The listing builds one solid part. Answer for the finished solid, in the listing's coordinates (mm). Face numbers are marked on the shaded views. A direction names the side the tool comes from. Round coordinates to 2 decimals unless told otherwise and drop trailing zeros. Order: outer loops, then holes, each group sorted by start corner. A loop starts at its lowest first (then second) coordinate and runs counter-clockwise, first axis right, second up. Notation, with made-up numbers: (-35, -0.75) - (-19, -0.75) arc R10 ccw to (-19, 18.25) - close; hole circle Ø10 at (-2, 44). An arc over 180 degrees is marked (long way). Use CSV: the item, a comma, the result in double quotes. Start each with the question number.
Item 1: For the marked faces 1, 2 and 3, determine the directions among +Z, -Z, +X, -X, +Y, -Y from which every point of the face is accessible in a straight line to the end or side of a thin tool.
Item 2: Find section A-A, the plane y = 1.6. Give the vertices of the cut face in (x, z) (3 decimals).
Item 3: Find section B-B, the plane x = 2.55. Count the separate pieces of the cut face and the enclosed holes in it, plus the area to 3 significant figures.
Item 4: A flat-ended cylindrical pin translates along its axis: P1, Ø1.1, axis at x = 0.5, y = -1, coming from the -Z side. Find the tip coordinate at first contact, or state that the pin passes through.
Item 5: Determine the mould class of the marked faces 4, 5, 6 and 7 for opening direction X: +X half, -X half, draft (parallel to the pull), parting line (faces both ways), or undercut.
Item 6: Straight lines are drawn through the part: line 1 along Y through (x, z) = (-0.1, 2.5); line 2 along X through (y, z) = (-1.2, 4.5) (3 decimals); line 3 along Z through (x, y) = (0.8, -2.15). For each, find the intervals that lie inside material, in ascending order. Write a range as [from, to].
Item 7: Find section C-C, the plane z = 3.25. Give the vertices of the cut face in (x, y) (3 decimals).
```python
from build123d import *

# Parameters (mm, degrees)
SKETCH006_W      = 1.85
SKETCH006_H      = 1.4
EXTRUDE006_DEPTH = 6.3
SKETCH007_W      = 1
SKETCH007_H      = 1
EXTRUDE007_DEPTH = 9
SKETCH010_W      = 4
SKETCH010_H      = 4
EXTRUDE010_DEPTH = 0.5
SKETCH011_W      = 3.2
SKETCH011_H      = 5
EXTRUDE011_DEPTH = 6.8
CHAMFER002_SIZE  = 0.4
ARRAY004_X_COUNT = 2
ARRAY004_X_PITCH = 2.54


with BuildPart() as extrude006:
    # Sketch006 → Extrude006 (new body)
    with BuildSketch(Plane.XY):
        Rectangle(SKETCH006_W, SKETCH006_H)
    extrude(amount=EXTRUDE006_DEPTH)


with BuildPart() as fusion004:
    # Sketch007 → Extrude007 (new body)
    with BuildSketch(Plane.XY):
        Rectangle(SKETCH007_W, SKETCH007_H)
    extrude(amount=EXTRUDE007_DEPTH)

    # Fusion004: union Extrude006
    add(extrude006.part)


with BuildPart() as fusion004_1:
    # Fusion004 placement: moved
    add(fusion004.part.moved(Location((0, 1.27, 0))))


with BuildPart() as extrude010:
    # Sketch010 → Extrude010 (new body)
    with BuildSketch(Plane.XY):
        Rectangle(SKETCH010_W, SKETCH010_H)
    extrude(amount=EXTRUDE010_DEPTH)


with BuildPart() as fusion005:
    # Part__Mirroring002: instance of Fusion004
    add(fusion004_1.part.mirror(Plane(origin=(0, 0, 0), x_dir=(1, 0, 0), z_dir=(0, 1, 0))))

    # Fusion005: union Fusion004, Extrude010
    add(fusion004_1.part)
    add(extrude010.part)


with BuildPart() as body002:
    # Sketch011 → Extrude011 (new body)
    with BuildSketch(Plane.XY):
        Rectangle(SKETCH011_W, SKETCH011_H)
    extrude(amount=EXTRUDE011_DEPTH)

    # Cut: cut Fusion005
    add(fusion005.part, mode=Mode.SUBTRACT)

    # Chamfer002
    chamfer002_edges = [body002.edges().sort_by_distance(p)[0] for p in [
        (0, -0.77, 6.8),
        (-0.5, -1.27, 6.8),
        (0, -1.77, 6.8),
        (0.5, -1.27, 6.8),
        (0.5, 1.27, 6.8),
        (0, 1.77, 6.8),
        (-0.5, 1.27, 6.8),
        (0, 0.77, 6.8),
    ]]
    chamfer(chamfer002_edges, length=CHAMFER002_SIZE)

    # Array004 X: body002 ×2


with BuildPart() as body002_1:
    add(body002.part)
    with Locations(*[(i * ARRAY004_X_PITCH, 0, 0) for i in range(1, ARRAY004_X_COUNT)]):
        add(body002.part)


solid = body002_1.part
```
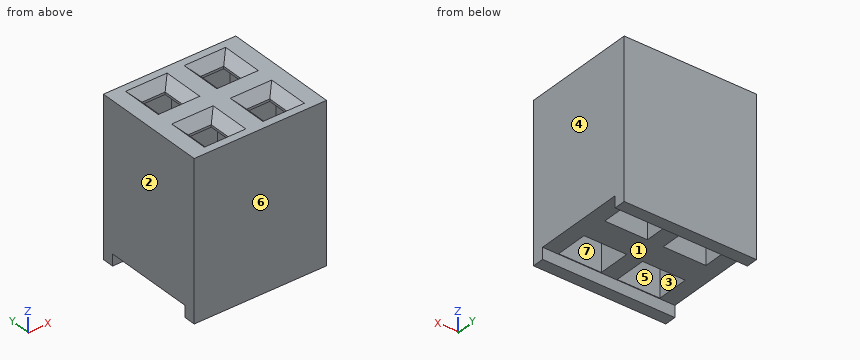
Worked out:
1,face 1,"-Z, +X, -X"
1,face 2,"+Z, -Z, -X, +Y, -Y"
1,face 3,"-Z"
2,outline,"(-1.6, 0.5) - (-0.925, 0.5) - (-0.925, 6.3) - (-0.5, 6.3) - (-0.5, 6.4) - (-0.9, 6.8) - (-1.6, 6.8) - close; (0.5, 6.3) - (0.925, 6.3) - (0.925, 0.5) - (1.615, 0.5) - (1.615, 6.3) - (2.04, 6.3) - (2.04, 6.4) - (1.64, 6.8) - (0.9, 6.8) - (0.5, 6.4) - close; (3.04, 6.3) - (3.465, 6.3) - (3.465, 0.5) - (4.14, 0.5) - (4.14, 6.8) - (3.44, 6.8) - (3.04, 6.4) - close"
3,separate pieces,"3"
3,enclosed holes,"0"
3,area,"14.4 mm²"
4,P1,"stops at z = 0.5"
5,face 4,"+X half"
5,face 5,"undercut"
5,face 6,"draft"
5,face 7,"undercut"
6,line 1,"y = [-2.5, -1.97], [-0.57, 0.57], [1.97, 2.5]"
6,line 2,"x = [-1.6, -0.925], [0.925, 1.615], [3.465, 4.14]"
6,line 3,"z = [0, 6.78]"
7,outline,"(-1.6, -2.5) - (4.14, -2.5) - (4.14, 2.5) - (-1.6, 2.5) - close; hole (-0.925, -1.97) - (0.925, -1.97) - (0.925, -0.57) - (-0.925, -0.57) - close; hole (-0.925, 0.57) - (0.925, 0.57) - (0.925, 1.97) - (-0.925, 1.97) - close; hole (1.615, -1.97) - (3.465, -1.97) - (3.465, -0.57) - (1.615, -0.57) - close; hole (1.615, 0.57) - (3.465, 0.57) - (3.465, 1.97) - (1.615, 1.97) - close"
